Can you work these out from the model? Positions are in its coordinate system, mm. A direction names the side the tool comes from. Coordinates: 2 decimals unless noted, no trailing zeros. Loops run counter-clockwise (first coordinate to the right, second up) from the corner with the lowest first, then second, coordinate; pieces in that order, holes last.
```python
from build123d import *

# Parameters (mm, degrees)
TORUS_R        = 1.5
CYLINDER_R     = 17
CYLINDER_DEPTH = 50
FILLET001_R    = 1
ARRAY_X_COUNT  = 2
ARRAY_X_PITCH  = 32
ARRAY_Y_COUNT  = 2
ARRAY_Y_PITCH  = 32
BOX_W          = 40
BOX_H          = 40
BOX_DEPTH      = 4
FILLET_R       = 1.5


with BuildPart() as part_cilindre:
    # Torus → Torus (revolve)
    with BuildSketch(Plane(origin=(0, 0, 50), x_dir=(1, 0, 0), z_dir=(0, -1, 0))):
        with Locations((12, 0)):
            Circle(TORUS_R)
    revolve(axis=Axis((0, 0, 50), (0, 0, 1)))


with BuildPart() as obj1:
    # Cylinder → Cylinder (new body)
    with BuildSketch(Plane.XY):
        Circle(CYLINDER_R)
    extrude(amount=CYLINDER_DEPTH)

    # Fillet001
    fillet001_edges = [obj1.edges().sort_by_distance(p)[0] for p in [
        (-17, 0, 50),
    ]]
    fillet(fillet001_edges, radius=FILLET001_R)

    # Cut001: cut part_cilindre
    add(part_cilindre.part, mode=Mode.SUBTRACT)


with BuildPart() as obj1_1:
    # Cut001 placement: moved
    add(obj1.part.moved(Location((20, 20, 4))))


with BuildPart() as array:
    # Sphere → Sphere (revolve)
    with BuildSketch(Plane(origin=(4, 4, 4), x_dir=(1, 0, 0), z_dir=(0, -1, 0))):
        with BuildLine():
            ThreePointArc((0, -2.4), (2.4, 0), (0, 2.4))
            Line((0, 2.4), (0, -2.4))
        make_face()
    revolve(axis=Axis((4, 4, 4), (0, 0, 1)))

    # Array X: Array ×2


with BuildPart() as array_1:
    add(array.part)
    with Locations(*[(i * ARRAY_X_PITCH, 0, 0) for i in range(1, ARRAY_X_COUNT)]):
        add(array.part)

    # Array Y: Array ×2


with BuildPart() as array_2:
    add(array_1.part)
    with Locations(*[(0, i * ARRAY_Y_PITCH, 0) for i in range(1, ARRAY_Y_COUNT)]):
        add(array_1.part)


with BuildPart() as obj2:
    # Box → Box (new body)
    with BuildSketch(Plane.XY):
        with Locations((20, 20)):
            Rectangle(BOX_W, BOX_H)
    extrude(amount=BOX_DEPTH)

    # Fillet
    fillet_edges = [obj2.edges().sort_by_distance(p)[0] for p in [
        (0, 0, 2),
        (0, 40, 2),
        (40, 0, 2),
        (40, 40, 2),
    ]]
    fillet(fillet_edges, radius=FILLET_R)

    # Cut: cut Array
    add(array_2.part, mode=Mode.SUBTRACT)

    # Fusion: union obj1
    add(obj1_1.part)


solid = obj2.part
```
(1) I want a section at C-C on z = 39. Write out the boundary of the cut face in (x, y), then the cut area to 3 significant figures.
Check values:
outline: circle Ø34 at (20, 20)
area: 908 mm2
(2) Which directions (+Z, -Z, +X, -X, +Y, -Y) give clear straight access to the entire face, cutting with the end or side of a thin tool? Please do faces 1 (the cylindrical face through (0.43, 0.45, 2.03)), 2 (the flat face through (2, 20, 4)).
Check values:
face 1: +Z, -Z, -X, -Y
face 2: +Z
(3) If I drill on probe 1 along Z at (x, y) = (2.5, 32); probe 2 along Z at (x, y) = (31, 16); probe 3 along Y at (x, z) = (22.5, 17.5), over which ranges is the centre line in solid material (lowest first)?
Check values:
probe 1: z = 0 to 4
probe 2: z = 0 to 52.53
probe 3: y = 3.18 to 36.82
(4) I'm going to push flat-ended pins straight in: pin 1 (6 mm diameter, centred on x = 17.5, z = 43, fed in from +Y); pin 2 (2 mm diameter, centred on x = 18, z = 10.5, fed in from -Y); pin 3 (1 mm diameter, centred on y = 32, z = 43, fed in from -X). Where does each tip first touch, or does it pass through?
Check values:
pin 1: stops at y = 37
pin 2: stops at y = 3.03
pin 3: stops at x = 7.48
(5) I want a section at A-A on y = 20. Write out the boundary of the cut face in (x, z).
Check values:
outline: (0, 0) - (40, 0) - (40, 4) - (37, 4) - (37, 53) arc R1 ccw to (36, 54) - (33.5, 54) arc R1.5 cw to (30.5, 54) - (9.5, 54) arc R1.5 cw to (6.5, 54) - (4, 54) arc R1 ccw to (3, 53) - (3, 4) - (0, 4) - close
